```python
from build123d import *

# Parameters (mm, degrees)
SKETCH1_W           = 25.4
SKETCH1_H           = 25.4
BOSS_EXTRUDE1_DEPTH = 367.12
CUT_EXTRUDE1_DEPTH  = 380
CUT_EXTRUDE2_DEPTH  = 380
SHELL1_T            = -1.651


with BuildPart() as part:
    # Sketch1 → Boss-Extrude1 (new body)
    with BuildSketch(Plane.XY):
        with Locations((12.7, 12.7)):
            Rectangle(SKETCH1_W, SKETCH1_H)
    extrude(amount=BOSS_EXTRUDE1_DEPTH)

    # Sketch2 → Cut-Extrude1 (cut)
    with BuildSketch(Plane(origin=(0, 25.4, 0), x_dir=(1, 0, 0), z_dir=(0, 1, 0))):
        Polygon((0, 0), (25.4, -37.855551052), (25.4, 0), align=None)
    extrude(amount=-CUT_EXTRUDE1_DEPTH, mode=Mode.SUBTRACT)

    # Sketch3 → Cut-Extrude2 (cut)
    with BuildSketch(Plane(origin=(0, 25.4, 0), x_dir=(1, 0, 0), z_dir=(0, 1, 0))):
        Polygon((0, -367.12), (25.4, -338.043933141), (25.4, -367.12), align=None)
    extrude(amount=-CUT_EXTRUDE2_DEPTH, mode=Mode.SUBTRACT)

    # Shell1
    shell1_openings = [part.faces().sort_by_distance(p)[0] for p in [
        (12.7, 12.7, 18.927775526),
        (12.7, 12.7, 352.58196657),
    ]]
    offset(amount=SHELL1_T, openings=shell1_openings, kind=Kind.INTERSECTION)


solid = part.part
```
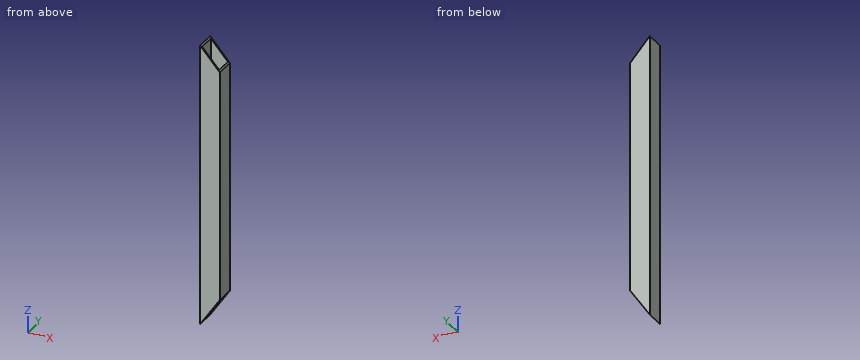
Design review of the part built by this model. Coordinates are the model's own, in mm. Round coordinates to 2 decimals unless told otherwise and drop trailing zeros. Write each loop counter-clockwise with the first axis right and the second up, starting at its lowest first coordinate (ties: lowest second). Pieces come first, ordered by that corner, then holes.
Item 1: We need section B-B on x = 17.5. Write out the cut boundary in (y, z).
Item 2: For probe 1 along Y at (x, z) = (20.25, 114.5); probe 2 along X at (y, z) = (18, 23), list the stretches that pass through material, from the lowest coordinate up.
Item 3: Clearance check with flat-ended pins moving along their axes: pin 1 Ø11 at (y, z) = (9.5, 125) entering from -X; pin 2 Ø12 at (x, y) = (11, 8.5) entering from -Z; pin 3 Ø6 at (x, y) = (17, 3) entering from -Z; pin 4 Ø6 at (x, y) = (22.5, 9) entering from -Z. State where each tip first meets the part, or that it passes through.
Item 4: We need section C-C on z = 152. Write out the cut boundary in (x, y).
Item 5: We need section A-A on y = 20.75. Write out the cut boundary in (x, z), and give its area (3 significant figures).
Returned:
1. outline: (0, 26.08) - (1.65, 26.08) - (1.65, 347.09) - (0, 347.09) - close; (23.75, 26.08) - (25.4, 26.08) - (25.4, 347.09) - (23.75, 347.09) - close
2. probe 1: y = 0 to 1.65, 23.75 to 25.4
2. probe 2: x = 0 to 1.65
3. pin 1: stops at x = 0
3. pin 2: passes through
3. pin 3: stops at z = 21.34
3. pin 4: stops at z = 35.39
4. outline: (0, 0) - (25.4, 0) - (25.4, 25.4) - (0, 25.4) - close; hole (1.65, 1.65) - (23.75, 1.65) - (23.75, 23.75) - (1.65, 23.75) - close
5. outline: (0, 0) - (1.65, 2.46) - (1.65, 365.23) - (0, 367.12) - close; (23.75, 35.39) - (25.4, 37.86) - (25.4, 338.04) - (23.75, 339.93) - close
5. area: 1,100 mm2
